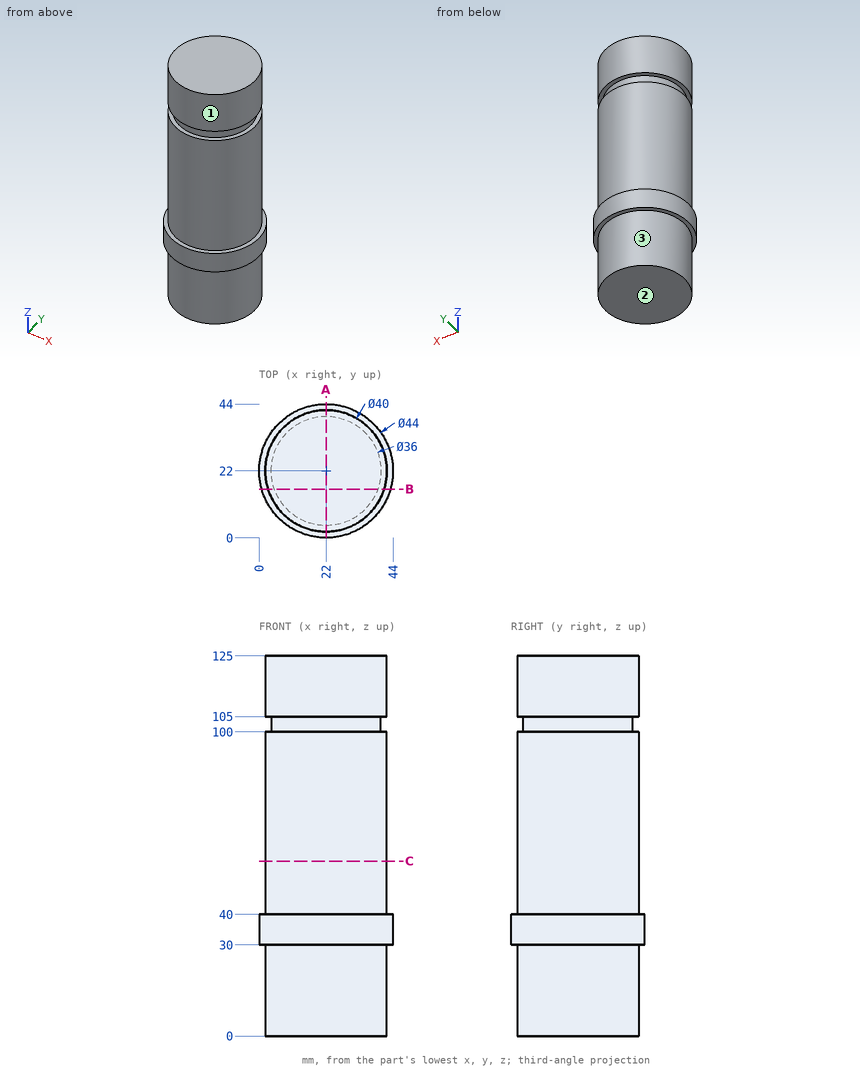
Check sheet for the drawn part. Datum: minimum x, y, z corner. Units: mm. A direction names the side the tool comes from. Coordinates: 2 decimals unless noted, no trailing zeros. Loops run counter-clockwise (first coordinate to the right, second up) from the corner with the lowest first, then second, coordinate; pieces in that order, holes last. Notation, with made-up numbers: (56.25, 64) - (101.25, 64) arc R17 ccw to (101.25, 93) - close; hole circle Ø3 at (-5, 77.5). An arc over 180 degrees is marked (long way). Put each result on its own line as item: value.
Item 1: Section check A-A (x = 22). Enter the section's corners in (y, z).
Conclusion:
outline: (0, 30) - (2, 30) - (2, 0) - (42, 0) - (42, 30) - (44, 30) - (44, 40) - (42, 40) - (42, 100) - (40, 100) - (40, 105) - (42, 105) - (42, 125) - (2, 125) - (2, 105) - (4, 105) - (4, 100) - (2, 100) - (2, 40) - (0, 40) - close
Item 2: Gauge pin test, flat ends, axial feed: pin 1 Ø5 at (x, z) = (29.5, 71.5) entering from -Y; pin 2 Ø10 at (x, z) = (19, 52.5) entering from -Y; pin 3 Ø10 at (y, z) = (24, 49.5) entering from -X. Record the tip position at first contact, or that the pin passes through.
Conclusion:
pin 1: stops at y = 2.64
pin 2: stops at y = 2
pin 3: stops at x = 2
Item 3: Scan lines: line 1 along Z through (x, y) = (12.5, 37.5); line 2 along X through (y, z) = (22.5, 49.5); line 3 along Z through (x, y) = (12, 3.5). Record each from-to range of solid material in increasing order.
Conclusion:
line 1: z = 0 to 100, 105 to 125
line 2: x = 2.01 to 41.99
line 3: z = 30 to 40
Item 4: Set-up check for the marked faces 1, 2 and 3: record each of +Z, -Z, +X, -X, +Y, -Y from which the full face is reachable in a straight line by a thin tool's end or side.
Conclusion:
face 1: +Z
face 2: -Z, +X, -X, +Y, -Y
face 3: -Z
Item 5: Section check B-B (y = 16). Enter the section's corners in (x, z).
Conclusion:
outline: (0.83, 30) - (2.92, 30) - (2.92, 0) - (41.08, 0) - (41.08, 30) - (43.17, 30) - (43.17, 40) - (41.08, 40) - (41.08, 100) - (38.97, 100) - (38.97, 105) - (41.08, 105) - (41.08, 125) - (2.92, 125) - (2.92, 105) - (5.03, 105) - (5.03, 100) - (2.92, 100) - (2.92, 40) - (0.83, 40) - close
Item 6: Section check C-C (z = 57.5). Enter the section's corners in (x, y).
Conclusion:
outline: circle Ø40 at (22, 22)
